Check sheet for the drawn part. Datum: minimum x, y, z corner. Units: mm. Give positions to 0.01 mm unless a question says otherwise; leave off trailing zeros. Order: outer loops, then holes, each group sorted by start corner. A loop starts at its lowest first (then second) coordinate and runs counter-clockwise, first axis right, second up. Notation, with made-up numbers: M 49.25,2.25 L 61.25,2.25 A22 ccw 61.25,24.25 Z; hole C 2.5,8 d8. An arc over 180 degrees is marked long. Answer in a Markdown table with one row per item. Add a question column.
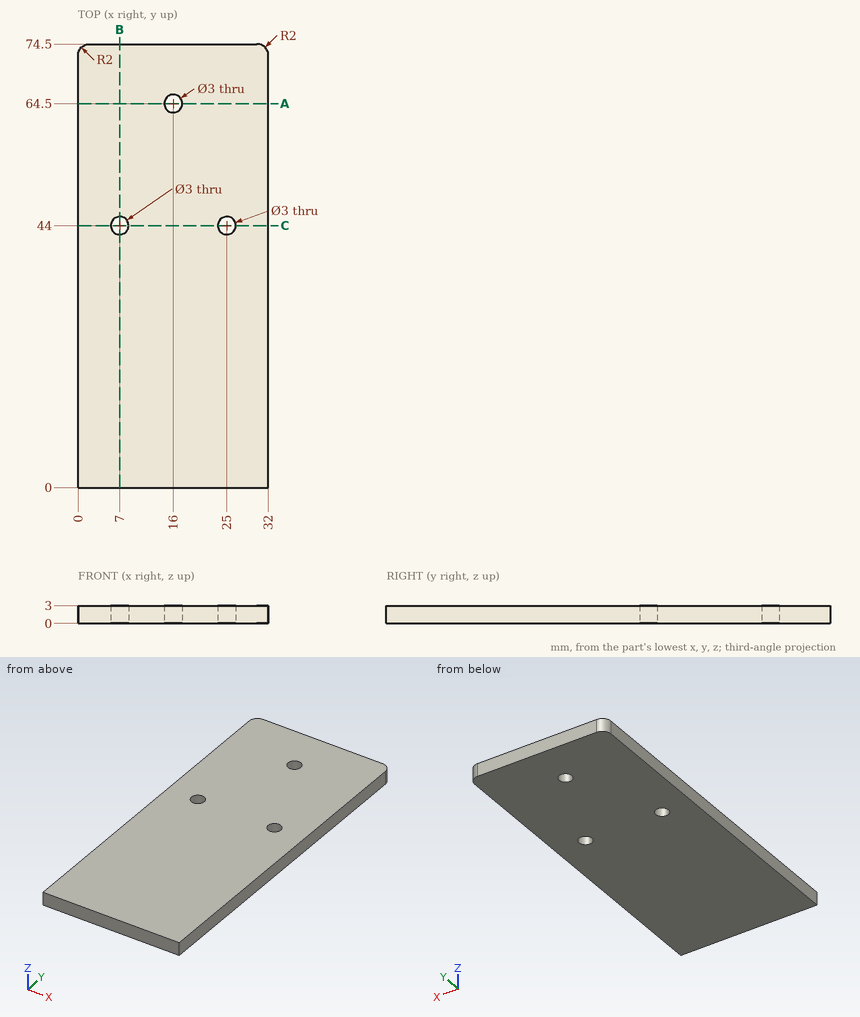
Q1. Cross-section at C-C (y = 44). Record the boundary of the cut face in (x, z), and give its area (3 significant figures).
Q2. Go/stop test with a flat-tipped pin: pin 1 (2.5 mm diameter, centred on x = 7, y = 44, fed in from -Z). Record where the tip stops, or that it passes through.
Q3. Thickness scan on probe 1 along Y at (x, z) = (16, 0.7); probe 2 along Y at (x, z) = (25, 0.6); probe 3 along X at (y, z) = (64.5, 2.3). Record the ranges inside material, lowest first.
Q4. Cross-section at A-A (y = 64.5). Record the boundary of the cut face in (x, z).
Q5. Cross-section at B-B (x = 7). Record the boundary of the cut face in (y, z), and give its area (4 significant figures).
Values follow:
| question | item | result |
|---|---|---|
| 1 | outline | M 0,0 L 5.5,0 L 5.5,3 L 0,3 Z; M 8.5,0 L 23.5,0 L 23.5,3 L 8.5,3 Z; M 26.5,0 L 32,0 L 32,3 L 26.5,3 Z |
| 1 | area | 78.0 mm² |
| 2 | pin 1 | through |
| 3 | probe 1 | 0 to 63, 66 to 74.5 |
| 3 | probe 2 | 0 to 42.5, 45.5 to 74.5 |
| 3 | probe 3 | 0 to 14.5, 17.5 to 32 |
| 4 | outline | M 0,0 L 14.5,0 L 14.5,3 L 0,3 Z; M 17.5,0 L 32,0 L 32,3 L 17.5,3 Z |
| 5 | outline | M 0,0 L 42.5,0 L 42.5,3 L 0,3 Z; M 45.5,0 L 74.5,0 L 74.5,3 L 45.5,3 Z |
| 5 | area | 214.5 mm² |
